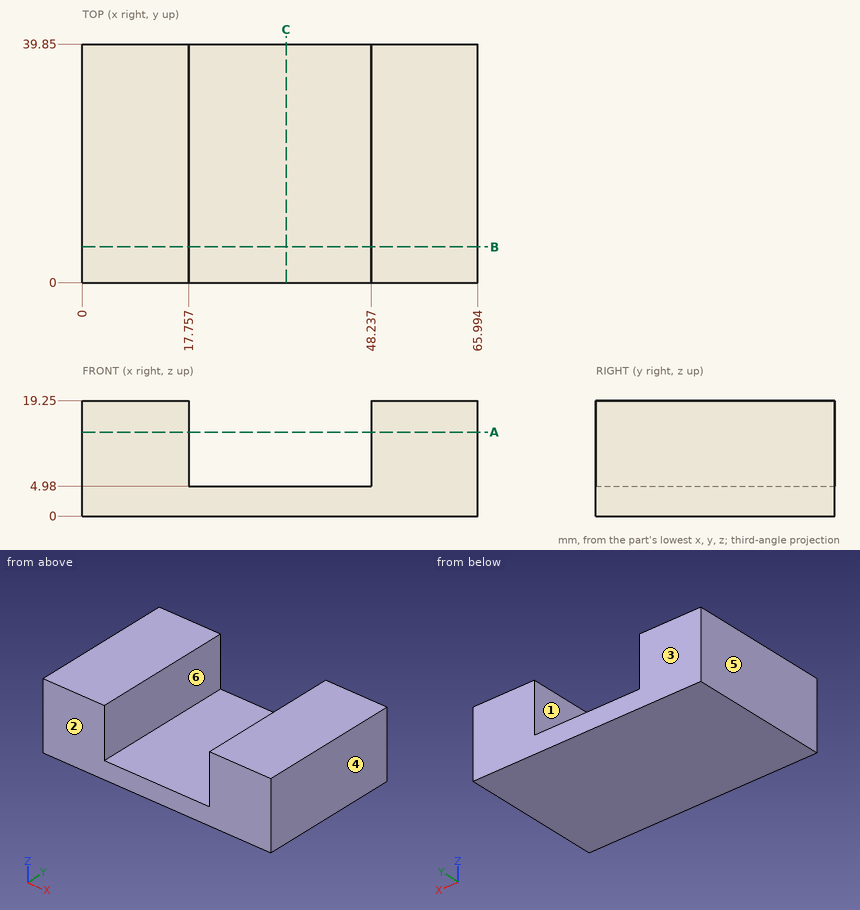
Check sheet for the drawn part. Datum: minimum x, y, z corner. Units: mm. A direction names the side the tool comes from. Coordinates: 2 decimals unless noted, no trailing zeros. Loops run counter-clockwise (first coordinate to the right, second up) from the corner with the lowest first, then second, coordinate; pieces in that order, holes last. Notation, with made-up numbers: (37, -30.75) -> (62, -30.75) arc R10 cw to (62, -24.75) -> close; hole circle Ø11 at (-23, 58). An arc over 180 degrees is marked (long way). Answer as a JSON object with one key per item and string values. Group by question number.
Item 1: Sectioned sample at C-C on x = 34. Record the boundary of the cut face in (y, z), plus the area to 3 significant figures.
Item 2: Scan lines: probe 1 along X at (y, z) = (35, 14.75); probe 2 along Z at (x, y) = (19, 29.5). Record each from-to range of solid material in increasing order.
Item 3: Depth check by flat-ended pin: pin 1 (1.5 mm diameter, centred on x = 21, y = 6, fed in from +Z). Enter the tip coordinate at first touch or a pass-through.
Item 4: Mould release check, pull along X, two halves, no side actions. Record for the marked faces 3, 4, 5 and 6: +X half, -X half, draft (parallel to the pull), parting line (faces both ways), or undercut.
Item 5: Tool access check on the marked faces 1 and 2. Record the directions out of +Z, -Z, +X, -X, +Y, -Y that give a thin tool (end or side, any length) a straight path to the whole face; none if there is none.
Item 6: Sectioned sample at A-A on z = 14. Record the boundary of the cut face in (x, y), plus the area to 3 significant figures.
Item 7: Sectioned sample at B-B on y = 6. Record the boundary of the cut face in (x, z).
Evaluation:
{
 "1": {"outline": "(0, 0) -> (39.85, 0) -> (39.85, 4.98) -> (0, 4.98) -> close", "area": "198 mm²"},
 "2": {"probe 1": "x = 0 to 17.76, 48.24 to 65.99", "probe 2": "z = 0 to 4.98"},
 "3": {"pin 1": "stops at z = 4.98"},
 "4": {"face 3": "draft", "face 4": "+X half", "face 5": "-X half", "face 6": "undercut"},
 "5": {"face 1": "+Z, +Y, -Y", "face 2": "+Z, -Z, +X, -X, -Y"},
 "6": {"outline": "(0, 0) -> (17.76, 0) -> (17.76, 39.85) -> (0, 39.85) -> close; (48.24, 0) -> (65.99, 0) -> (65.99, 39.85) -> (48.24, 39.85) -> close", "area": "1,420 mm²"},
 "7": {"outline": "(0, 0) -> (65.99, 0) -> (65.99, 19.25) -> (48.24, 19.25) -> (48.24, 4.98) -> (17.76, 4.98) -> (17.76, 19.25) -> (0, 19.25) -> close"}
}
